For this review, take the finished solid that the model builds, in its own axes (mm). A direction names the side the tool comes from. Coordinates: 2 decimals unless noted, no trailing zeros. Write each loop counter-clockwise with the first axis right and the second up, starting at its lowest first coordinate (ties: lowest second). Pieces come first, ordered by that corner, then holes.
```python
from build123d import *

# Parameters (mm, degrees)
F0_R     = 50.8
F1_DEPTH = 723.9
F3_DEPTH = 25.4
F4_R     = 12.7


with BuildPart() as f1:
    # F0 (on Top) → F1 (new body)
    with BuildSketch(Plane.XY):
        Circle(F0_R)
    extrude(amount=-F1_DEPTH)

    # F2 (on face) → F3 (join)
    with BuildSketch(Plane(origin=(0, 0, -723.9), x_dir=(1, 0, 0), z_dir=(0, 0, -1))):
        with BuildLine():
            Line((-228.996531, 202.055763), (-46.770065, 19.829297))
            ThreePointArc((-46.770065, 19.829297), (-35.921024, 35.921024), (-19.829297, 46.770065))
            Line((-19.829297, 46.770065), (-202.055763, 228.996531))
            Line((-202.055763, 228.996531), (-228.996531, 202.055763))
        make_face()
        with BuildLine():
            Line((202.055763, 228.996531), (19.829297, 46.770065))
            ThreePointArc((19.829297, 46.770065), (35.921024, 35.921024), (46.770065, 19.829297))
            Line((46.770065, 19.829297), (228.996531, 202.055763))
            Line((228.996531, 202.055763), (202.055763, 228.996531))
        make_face()
        with BuildLine():
            ThreePointArc((46.770065, -19.829297), (35.921024, -35.921024), (19.829297, -46.770065))
            Line((19.829297, -46.770065), (202.055763, -228.996531))
            Line((202.055763, -228.996531), (228.996531, -202.055763))
            Line((228.996531, -202.055763), (46.770065, -19.829297))
        make_face()
        with BuildLine():
            ThreePointArc((-19.829297, -46.770065), (-35.921024, -35.921024), (-46.770065, -19.829297))
            Line((-46.770065, -19.829297), (-228.996531, -202.055763))
            Line((-228.996531, -202.055763), (-202.055763, -228.996531))
            Line((-202.055763, -228.996531), (-19.829297, -46.770065))
        make_face()
    extrude(amount=-F3_DEPTH)

    # F4
    f4_edges = [f1.edges().sort_by_distance(p)[0] for p in [
        (-110.94253, -137.883298, -698.5),
        (-215.526147, -215.526147, -698.5),
        (-137.883298, -110.94253, -698.5),
        (-137.883298, 110.94253, -698.5),
        (-215.526147, 215.526147, -698.5),
        (-110.94253, 137.883298, -698.5),
        (110.94253, 137.883298, -698.5),
        (137.883298, 110.94253, -698.5),
        (215.526147, 215.526147, -698.5),
        (137.883298, -110.94253, -698.5),
        (110.94253, -137.883298, -698.5),
        (215.526147, -215.526147, -698.5),
    ]]
    fillet(f4_edges, radius=F4_R)


with BuildPart() as f5_1:
    # F5: copy of F1
    add(f1.part)


solid = f1.part
```
Q1. Clearance check with flat-ended pins moving along their axes: pin 1 Ø2 at (x, y) = (60.5, -73) entering from +Z; pin 2 Ø6 at (x, z) = (-35, -217.5) entering from -Y; pin 3 Ø4 at (x, z) = (-5, -79) entering from -Y. State where each tip first meets the part, or that it passes through.
Ans:
pin 1: stops at z = -698.59
pin 2: stops at y = -39.45
pin 3: stops at y = -50.71
Q2. Add section C-C (z = -551). State the section outline as (x, y) points, then the cut area to 3 significant figures.
Ans:
outline: circle Ø101.6 at (0, 0)
area: 8,110 mm2
Q3. Add section A-A (y = 0). State the section outline as (x, z) points, then the cut area to 3 significant figures.
Ans:
outline: (-50.8, -723.9) - (50.8, -723.9) - (50.8, 0) - (-50.8, 0) - close
area: 73,500 mm2
Q4. Tool access review of faces 4 (the flat face through (136.61, -109.67, -717.64)), 5 (the cylindrical face through (-136.6, 114.78, -702.32)), 6 (the flat face through (109.67, 136.61, -717.64)): name each direction out of +Z, -Z, +X, -X, +Y, -Y from which nothing blocks a thin tool from reaching the whole face with its end or side.
Ans:
face 4: +Z, -Z, +X
face 5: +Z, -X
face 6: +Z, -Z, +Y
Q5. Draft analysis for pull direction X (two halves, no side actions). For faces 1 (the flat face through (-112.22, 139.16, -717.64)), 2 (the flat face through (-139.16, -112.22, -717.64)), 3 (the flat face through (139.16, 112.22, -717.64)), state which applies: +X half, -X half, draft (parallel to the pull), parting line (faces both ways), or undercut.
Ans:
face 1: undercut
face 2: -X half
face 3: +X half
Q6. For probe 1 along Y at (x, z) = (2.5, -87); probe 2 along X at (y, z) = (-3.5, -550.5); probe 3 along X at (y, z) = (31, -112.5), list the stretches that pass through material, from the lowest coordinate up.
Ans:
probe 1: y = -50.74 to 50.74
probe 2: x = -50.68 to 50.68
probe 3: x = -40.24 to 40.24
